```python
from build123d import *

# Parameters (mm, degrees)
F0_W     = 10.65
F0_H     = 10.7820915088
F0_H_2   = 10.5179084912
F1_DEPTH = 35
F5_R     = 3.7
F6_DEPTH = 25
F7_R     = 3.7
F8_DEPTH = 25


with BuildPart() as f1:
    # F0 (on Top) → F1 (new body)
    with BuildSketch(Plane.XY):
        with Locations((-5.325, 15.9089542456)):
            Rectangle(F0_W, F0_H)
        with Locations((5.325, 15.9089542456)):
            Rectangle(F0_W, F0_H)
        with BuildLine():
            Line((28.999999983, 21.3), (10.65, 21.3))
            Line((10.65, 21.3), (10.65, 10.5179084912))
            Line((10.65, 10.5179084912), (18.3508191943, 10.5179084912))
            ThreePointArc((18.3508191943, 10.5179084912), (21.4227552913, 18.1338400989), (28.999999983, 21.3))
        make_face()
        with BuildLine():
            Line((39.65, 21.3), (28.999999983, 21.3))
            ThreePointArc((28.999999983, 21.3), (36.5306872136, 18.1806872257), (39.65, 10.65))
            Line((39.65, 10.65), (39.65, 21.3))
        make_face()
        with BuildLine():
            Line((39.65, 0), (39.65, 10.65))
            ThreePointArc((39.65, 10.65), (36.5306872196, 3.1193127804), (29, 0))
            Line((29, 0), (39.65, 0))
        make_face()
        with BuildLine():
            Line((18.3508191943, 10.5179084912), (10.65, 10.5179084912))
            Line((10.65, 10.5179084912), (10.65, 0))
            Line((10.65, 0), (29, 0))
            ThreePointArc((29, 0), (21.5161598951, 3.0727552973), (18.3508191943, 10.5179084912))
        make_face()
        with Locations((5.325, 5.2589542456)):
            Rectangle(F0_W, F0_H_2)
        with Locations((-5.325, 5.2589542456)):
            Rectangle(F0_W, F0_H_2)
        with BuildLine():
            Line((0, 0), (-10.65, 0))
            Line((-10.65, 0), (-10.65, -18.3500000446))
            ThreePointArc((-10.65, -18.3500000446), (-7.5306872354, -10.8193127961), (0, -7.7))
            Line((0, -7.7), (0, 0))
        make_face()
        with BuildLine():
            Line((10.65, 0), (0, 0))
            Line((0, 0), (0, -7.7))
            ThreePointArc((0, -7.7), (7.5306872196, -10.8193127804), (10.65, -18.35))
            Line((10.65, -18.35), (10.65, 0))
        make_face()
        with BuildLine():
            ThreePointArc((0, -29), (-7.5306872039, -25.8806872354), (-10.65, -18.3500000446))
            Line((-10.65, -18.3500000446), (-10.65, -29))
            Line((-10.65, -29), (0, -29))
        make_face()
        with BuildLine():
            ThreePointArc((10.65, -18.35), (7.5306872196, -25.8806872196), (0, -29))
            Line((0, -29), (10.65, -29))
            Line((10.65, -29), (10.65, -18.35))
        make_face()
        with BuildLine():
            ThreePointArc((0, -7.7), (-7.5306872354, -10.8193127961), (-10.65, -18.3500000446))
            ThreePointArc((-10.65, -18.3500000446), (-7.5306872039, -25.8806872354), (0, -29))
            ThreePointArc((0, -29), (7.5306872196, -25.8806872196), (10.65, -18.35))
            ThreePointArc((10.65, -18.35), (7.5306872196, -10.8193127804), (0, -7.7))
        make_face()
        with BuildLine():
            ThreePointArc((39.65, 10.65), (36.5306872136, 18.1806872257), (28.999999983, 21.3))
            ThreePointArc((28.999999983, 21.3), (21.4227552913, 18.1338400989), (18.3508191943, 10.5179084912))
            ThreePointArc((18.3508191943, 10.5179084912), (21.5161598951, 3.0727552973), (29, 0))
            ThreePointArc((29, 0), (36.5306872196, 3.1193127804), (39.65, 10.65))
        make_face()
    extrude(amount=F1_DEPTH)

    # F2 (on Right) → F3 (revolve, cut)
    with BuildSketch(Plane.YZ):
        with BuildLine():
            Line((-18.35, 0), (-18.35, 8.7915472686))
            ThreePointArc((-18.35, 8.7915472686), (-24.8692408708, 5.8217661701), (-29.0438234806, 0))
            Line((-29.0438234806, 0), (-18.35, 0))
        make_face()
    revolve(axis=Axis((0, -18.35, 6.2414296837), (0, 0, 1)), mode=Mode.SUBTRACT)

    # F5 (on Top) → F6 (cut)
    with BuildSketch(Plane.XY):
        with Locations((0, -18.35)):
            Circle(F5_R)
    extrude(amount=F6_DEPTH, mode=Mode.SUBTRACT)

    # F7 (on Top) → F8 (cut)
    with BuildSketch(Plane.XY):
        with Locations((29.1118938476, 10.736274533)):
            Circle(F7_R)
    extrude(amount=F8_DEPTH, mode=Mode.SUBTRACT)

    # F9 (on offset) → F10 (revolve, cut)
    with BuildSketch(Plane.XZ.offset(-10.65)):
        with BuildLine():
            Line((18.3073151857, 0), (28.9965979755, 0))
            Line((28.9965979755, 0), (28.9965979755, 9.6057383344))
            ThreePointArc((28.9965979755, 9.6057383344), (22.567565814, 6.0095811507), (18.3073151857, 0))
        make_face()
    revolve(axis=Axis((28.9965979755, 10.65, 11.7063857615), (0, 0, 1)), mode=Mode.SUBTRACT)


solid = f1.part
```
Can you work these out from the model? Positions are in its coordinate system, mm. A direction names the side the tool comes from. Give positions to 0.01 mm unless a question says otherwise; leave off trailing zeros. Loops run counter-clockwise (first coordinate to the right, second up) from the corner with the lowest first, then second, coordinate; pieces in that order, holes last. Notation, with made-up numbers: M 52,-39.5 L 94,-39.5 A28 ccw 94,-1.5 Z; hole C 2.5,32 d1. An arc over 180 degrees is marked long. Use one line per item in the form item = value. Start each with the question number.
(1) Thinking about a two-plate mould opening in X: for faces 1 (the flat face through (-10.65, -3, 17)), 2 (the cylindrical face through (25.415, 10.899, 16.339)), 3 (the flat face through (9, 2, 35)), which applies, released by +X, released by -X, zero draft, split by the parting line, or undercut?
(2) Please list where these lines run through material, in increasing order: line 1 (X direction, y = -18, z = 15.5); line 2 (X direction, y = -9, z = 13); line 3 (Y direction, x = 28.5, z = 29).
(3) On a 3-axis mill with a long thin cutter (end or side, diameter ignored), from which of +Z, -Z, +X, -X, +Y, -Y can I reach the whole of each face in a straight line? I mean faces 4 (the flat face through (29, 11, 25)), 5 (the flat face through (15, 21.3, 17)), 6 (the flat face through (25, 0, 17)). Say none if no direction works.
(4) I want a section at A-A, the plane z = 11. Write out the boundary of the cut face in (x, y).
(5) I want a section at B-B, the plane z = 31.5. Write out the boundary of the cut face in (x, y).
(6) I'm going to push flat-ended pins straight in: P1, Ø14.5, axis at x = 31, z = 17, coming from the -Y side; P2, Ø3.5, axis at x = 1, y = -17, coming from the -Z side; P3, Ø6, axis at x = 30.5, y = 11.5, coming from the -Z side. Where does each tip first touch, or does it pass through?
Worked out:
q1.face_1 = released by -X
q1.face_2 = undercut
q1.face_3 = zero draft
q2.line_1 = -10.65 to -3.68, 3.68 to 10.65
q2.line_2 = -10.65 to 10.65
q2.line_3 = 0 to 21.3
q3.face_4 = -Z
q3.face_5 = +Z, -Z, +X, -X, +Y
q3.face_6 = +Z, -Z, +X, -Y
q4.outline = M -10.65,-29 L 10.65,-29 L 10.65,0 L 39.65,0 L 39.65,21.3 L -10.65,21.3 Z; hole C 0,-18.35 d7.4; hole C 29.11,10.74 d7.4
q5.outline = M -10.65,-29 L 10.65,-29 L 10.65,0 L 39.65,0 L 39.65,21.3 L -10.65,21.3 Z
q6.P1 = 0
q6.P2 = 25
q6.P3 = 7.35
